from build123d import *

# Parameters (mm, degrees)
SALIENTE_EXTRUIR1_DEPTH = 350
CROQUIS2_R              = 4.7625
CORTAR_EXTRUIR1_DEPTH   = 26.4


with BuildPart() as part:
    # Croquis1 → Saliente-Extruir1 (new body)
    with BuildSketch(Plane.XY):
        with BuildLine():
            Line((-10.2, -12.7), (10.2, -12.7))
            ThreePointArc((10.2, -12.7), (11.967766953, -11.967766953), (12.7, -10.2))
            Line((12.7, -10.2), (12.7, 10.2))
            ThreePointArc((12.7, 10.2), (11.967766953, 11.967766953), (10.2, 12.7))
            Line((10.2, 12.7), (-10.2, 12.7))
            ThreePointArc((-10.2, 12.7), (-11.967766953, 11.967766953), (-12.7, 10.2))
            Line((-12.7, 10.2), (-12.7, -10.2))
            ThreePointArc((-12.7, -10.2), (-11.967766953, -11.967766953), (-10.2, -12.7))
        make_face()
        with BuildLine():
            Line((-7.025, -9.525), (7.025, -9.525))
            ThreePointArc((7.025, -9.525), (8.792766953, -8.792766953), (9.525, -7.025))
            Line((9.525, -7.025), (9.525, 7.025))
            ThreePointArc((9.525, 7.025), (8.792766953, 8.792766953), (7.025, 9.525))
            Line((7.025, 9.525), (-7.025, 9.525))
            ThreePointArc((-7.025, 9.525), (-8.792766953, 8.792766953), (-9.525, 7.025))
            Line((-9.525, 7.025), (-9.525, -7.025))
            ThreePointArc((-9.525, -7.025), (-8.792766953, -8.792766953), (-7.025, -9.525))
        make_face(mode=Mode.SUBTRACT)
    extrude(amount=SALIENTE_EXTRUIR1_DEPTH)

    # Croquis2 → Cortar-Extruir1 (cut, through all)
    with BuildSketch(Plane.ZY.offset(12.7)):
        with Locations((50, 0)):
            Circle(CROQUIS2_R)
        with Locations((150, 0)):
            Circle(CROQUIS2_R)
    extrude(amount=-CORTAR_EXTRUIR1_DEPTH, mode=Mode.SUBTRACT)


solid = part.part
The model under review builds one solid part; all positions refer to its coordinate system, in mm. A direction names the side the tool comes from. Round coordinates to 2 decimals unless told otherwise and drop trailing zeros. Loops run counter-clockwise (first coordinate to the right, second up) from the corner with the lowest first, then second, coordinate; pieces in that order, holes last. Notation, with made-up numbers: (-14, 51) - (32, 51) arc R17 cw to (32, 60) - close; hole circle Ø8 at (-3.75, 33.25). An arc over 180 degrees is marked (long way). Use CSV: the item, a comma, the result in double quotes.
(1) The part is to be moulded in two halves that separate along Y. For faces 3 (the flat face through (0, -12.7, 173)), 4 (the flat face through (0, 12.7, 173)), 5 (the cylindrical face through (11.09, -1.82, 154.4)), say which applies: pulls with the +Y half, pulls with the -Y half, needs draft (parallel to the pull), parting line crosses it, or undercut.
Working result:
face 3,"pulls with the -Y half"
face 4,"pulls with the +Y half"
face 5,"undercut"
(2) Machinability: for faces 1 (the cylindrical face through (-11.13, -1.82, 154.4)), 2 (the flat face through (0, 9.525, 173)), which of the approach directions +Z, -Z, +X, -X, +Y, -Y give a long, thin tool a straight path to every point of the face, cutting with its end or side? Answer none if there is none.
Working result:
face 1,"+X, -X"
face 2,"+Z, -Z"
(3) Take a section at A-A, the plane y = 0. Give the boundary of the cut face in (x, z) (1 decimal), plus the area to 3 significant figures.
Working result:
outline,"(-12.7, 0) - (-9.5, 0) - (-9.5, 45.2) - (-12.7, 45.2) - close; (-12.7, 54.8) - (-9.5, 54.8) - (-9.5, 145.2) - (-12.7, 145.2) - close; (-12.7, 154.8) - (-9.5, 154.8) - (-9.5, 350) - (-12.7, 350) - close; (9.5, 0) - (12.7, 0) - (12.7, 45.2) - (9.5, 45.2) - close; (9.5, 54.8) - (12.7, 54.8) - (12.7, 145.2) - (9.5, 145.2) - close; (9.5, 154.8) - (12.7, 154.8) - (12.7, 350) - (9.5, 350) - close"
area,"2,100 mm^2"
(4) Take a section at D-D, the plane z = 150. Give the boundary of the cut face in (x, y) (1 decimal), plus the area to 3 significant figures.
Working result:
outline,"(-12.7, -10.2) arc R2.5 ccw to (-10.2, -12.7) - (10.2, -12.7) arc R2.5 ccw to (12.7, -10.2) - (12.7, -4.8) - (9.5, -4.8) - (9.5, -7) arc R2.5 cw to (7, -9.5) - (-7, -9.5) arc R2.5 cw to (-9.5, -7) - (-9.5, -4.8) - (-12.7, -4.8) - close; (-12.7, 4.8) - (-9.5, 4.8) - (-9.5, 7) arc R2.5 cw to (-7, 9.5) - (7, 9.5) arc R2.5 cw to (9.5, 7) - (9.5, 4.8) - (12.7, 4.8) - (12.7, 10.2) arc R2.5 ccw to (10.2, 12.7) - (-10.2, 12.7) arc R2.5 ccw to (-12.7, 10.2) - close"
area,"222 mm^2"
(5) Clearance check with a flat-ended pin moving along its axis: P1, Ø11, axis at y = 0, z = 50, coming from the -X side. State where the tip first meets the part, or that it passes through.
Working result:
P1,"stops at x = -12.7"
(6) Take a section at C-C, the plane z = 249. Give the boundary of the cut face in (x, y) (3 decimals), plus the area to 3 significant figures.
Working result:
outline,"(-12.7, -10.2) arc R2.5 ccw to (-10.2, -12.7) - (10.2, -12.7) arc R2.5 ccw to (12.7, -10.2) - (12.7, 10.2) arc R2.5 ccw to (10.2, 12.7) - (-10.2, 12.7) arc R2.5 ccw to (-12.7, 10.2) - close; hole (-9.525, -7.025) arc R2.5 ccw to (-7.025, -9.525) - (7.025, -9.525) arc R2.5 ccw to (9.525, -7.025) - (9.525, 7.025) arc R2.5 ccw to (7.025, 9.525) - (-7.025, 9.525) arc R2.5 ccw to (-9.525, 7.025) - close"
area,"282 mm^2"
(7) Take a section at B-B, the plane x = 4. Give the boundary of the cut face in (y, z) (3 decimals).
Working result:
outline,"(-12.7, 0) - (-9.525, 0) - (-9.525, 350) - (-12.7, 350) - close; (9.525, 0) - (12.7, 0) - (12.7, 350) - (9.525, 350) - close"
(8) For line 1 (Y direction, x = 0.5, z = 296) (3 decimals); line 2 (Y direction, x = -10.45, z = 150), list the stretches that pass through material, from the lowest coordinate up.
Working result:
line 1,"y = -12.7 to -9.525, 9.525 to 12.7"
line 2,"y = -12.69 to -4.76, 4.76 to 12.69"
